```python
from build123d import *

# Parameters (mm, degrees)
BOSS_EXTRUDE1_DEPTH = 5
FILLET1_R           = 5
FILLET3_R           = 5
FILLET4_R           = 5


with BuildPart() as part:
    # Sketch1 → Boss-Extrude1 (new body)
    with BuildSketch(Plane.XY):
        with BuildLine():
            Line((-108.310248072, -37.693381192), (-108.310248072, -19.713755061))
            Line((-108.310248072, -19.713755061), (76.399052405, -19.713755061))
            ThreePointArc((76.399052405, -19.713755061), (79.934586311, -18.249288967), (81.399052405, -14.713755061))
            Line((81.399052405, -14.713755061), (81.399052405, 89.326992678))
            ThreePointArc((81.399052405, 89.326992678), (79.934586311, 92.862526584), (76.399052405, 94.326992678))
            Line((76.399052405, 94.326992678), (-108.310248072, 94.326992678))
            Line((-108.310248072, 94.326992678), (-108.310248072, 112.306618808))
            ThreePointArc((-108.310248072, 112.306618808), (-122.452383696, 106.448754432), (-128.310248072, 92.306618808))
            Line((-128.310248072, 92.306618808), (-128.310248072, -17.693381192))
            ThreePointArc((-128.310248072, -17.693381192), (-122.452383696, -31.835516815), (-108.310248072, -37.693381192))
        make_face()
    extrude(amount=BOSS_EXTRUDE1_DEPTH)

    # Fillet1
    fillet1_edges = [part.edges().sort_by_distance(p)[0] for p in [
        (-15.955597834, -19.713755061, 0),
        (79.934586311, -18.249288967, 0),
        (81.399052405, 37.306618808, 0),
        (79.934586311, 92.862526584, 0),
        (-15.955597834, 94.326992678, 0),
    ]]
    fillet(fillet1_edges, radius=FILLET1_R - 0.0001)  # a hair under: the kernel refuses the full size

    # Fillet3
    fillet3_edges = [part.edges().sort_by_distance(p)[0] for p in [
        (-108.310248072, 100.816855743, 0),
    ]]
    fillet(fillet3_edges, radius=FILLET3_R - 0.0001)  # a hair under: the kernel refuses the full size

    # Fillet4
    fillet4_edges = [part.edges().sort_by_distance(p)[0] for p in [
        (-108.310248072, -26.203618126, 0),
    ]]
    fillet(fillet4_edges, radius=FILLET4_R - 0.0001)  # a hair under: the kernel refuses the full size


solid = part.part
```
CAD build for the part. Positions are in the model's coordinates, mm. A direction names the side the tool comes from. Give positions to 0.01 mm unless a question says otherwise; leave off trailing zeros.
(1) Tool access for faces 1 (the cylindrical face through (-19.8, 92.9, 1.5)), 2 (the cylindrical face through (-109.74, -28.6, 1.5)), 3 (the flat face through (-128.31, 38, 2)): list every direction of +Z, -Z, +X, -X, +Y, -Y with a clear straight run to the whole face (end or side of a thin tool).
(2) Flat gauge pins, fed straight in: pin 1 (5 mm diameter, centred on x = -106.5, y = -22, fed in from -Z); pin 2 (3 mm diameter, centred on x = 21, z = 2, fed in from +Y). Where does each tip first touch, or does it go through?
(3) Drill centre lines: L1, parallel to Y at x = 59, z = 4.5; L2, parallel to X at y = 29, z = 4.75; L3, parallel to X at y = 51, z = 3.25. Where is each one in solid material? Low to high.
Results found:
1. face 1: -Z, +X, +Y
1. face 2: -Z, +X, -Y
1. face 3: +Z, -Z, -X, +Y, -Y
2. pin 1: stops at z = 2.47
2. pin 2: stops at y = 94.1
3. L1: y = -19.69 to 94.3
3. L2: x = -128.31 to 81.39
3. L3: x = -128.31 to 81.08
